Model file for the job. Use its own axes, mm. Give positions to 0.01 mm unless a question says otherwise; leave off trailing zeros. Order: outer loops, then holes, each group sorted by start corner. A loop starts at its lowest first (then second) coordinate and runs counter-clockwise, first axis right, second up. Notation, with made-up numbers: (24, 83) - (66, 83) arc R32 cw to (66, 118) - close; hole circle Ø8 at (79, -9). An arc over 180 degrees is marked (long way). Return JSON: item names as keys, results as strings. Group by question number.
from build123d import *

# Parameters (mm, degrees)
EXTRUDE_THIN2_DEPTH      = 2.25
EXTRUDE_THIN2_DEPTH_BACK = 2.25
SKETCH2_W                = 2.5
SKETCH2_H                = 0.8
EXTRUDE1_DEPTH           = 4
EXTRUDE1_DEPTH_BACK      = 4
S2D0010_W                = 0.5
S2D0010_H                = 2.5
EXTRUDE2_DEPTH           = 0.17
EXTRUDE_THIN3_DEPTH      = 0.5
EXTRUDE_THIN3_DEPTH_BACK = 0.5
FILLET1_R                = 0.15
FILLET2_R                = 0.49


with BuildPart() as part:
    # Sketch1 → Extrude-Thin2 (new body, two sides)
    with BuildSketch(Plane(origin=(0, 0, 0), x_dir=(0, -1, 0), z_dir=(1, 0, 0))) as extrude_thin2_sk:
        with BuildLine():
            Line((-3.4, -0.6), (-2.8, -0.6))
            ThreePointArc((-2.8, -0.6), (-2.693933983, -0.556066017), (-2.65, -0.45))
            Line((-2.65, -0.45), (-2.65, 0))
            Line((-2.65, 0), (2.65, 0))
            Line((2.65, 0), (2.65, -0.45))
            ThreePointArc((2.65, -0.45), (2.693933983, -0.556066017), (2.8, -0.6))
            Line((2.8, -0.6), (3.4, -0.6))
            Line((3.4, -0.6), (3.4, -0.5))
            Line((3.4, -0.5), (2.8, -0.5))
            ThreePointArc((2.8, -0.5), (2.764644661, -0.485355339), (2.75, -0.45))
            Line((2.75, -0.45), (2.75, 0.1))
            Line((2.75, 0.1), (-2.75, 0.1))
            Line((-2.75, 0.1), (-2.75, -0.45))
            ThreePointArc((-2.75, -0.45), (-2.764644661, -0.485355339), (-2.8, -0.5))
            Line((-2.8, -0.5), (-3.4, -0.5))
            Line((-3.4, -0.5), (-3.4, -0.6))
        make_face()
    extrude(amount=EXTRUDE_THIN2_DEPTH)
    extrude(extrude_thin2_sk.sketch, amount=-EXTRUDE_THIN2_DEPTH_BACK)

    # Sketch2 → Extrude1 (cut, two sides)
    with BuildSketch(Plane(origin=(0, 0, 0), x_dir=(-1, 0, 0), z_dir=(0, 1, 0))) as extrude1_sk:
        with Locations((0, 0.4)):
            Rectangle(SKETCH2_W, SKETCH2_H)
    extrude(amount=EXTRUDE1_DEPTH, mode=Mode.SUBTRACT)
    extrude(extrude1_sk.sketch, amount=-EXTRUDE1_DEPTH_BACK, mode=Mode.SUBTRACT)

    # S2D0010 → Extrude2 (cut)
    with BuildSketch(Plane(origin=(0, 0, 0), x_dir=(0, -1, 0), z_dir=(0, 0, 1))):
        with BuildLine():
            Line((1.25, 1), (-1.25, 1))
            ThreePointArc((-1.25, 1), (-2.25, 0), (-1.25, -1))
            Line((-1.25, -1), (1.25, -1))
            ThreePointArc((1.25, -1), (2.25, 0), (1.25, 1))
        make_face()
        with Locations((2.75, 0)):
            Rectangle(S2D0010_W, S2D0010_H)
        with Locations((-2.75, 0)):
            Rectangle(S2D0010_W, S2D0010_H)
    extrude(amount=-EXTRUDE2_DEPTH, mode=Mode.SUBTRACT)

    # S2D0012 → Extrude-Thin3 (add, two sides)
    with BuildSketch(Plane(origin=(0, 0, 0), x_dir=(1, 0, 0), z_dir=(0, 1, 0))) as extrude_thin3_sk:
        with BuildLine():
            Line((2.25, 0), (2.45, 0))
            ThreePointArc((2.45, 0), (2.485355339, -0.014644661), (2.5, -0.05))
            Line((2.5, -0.05), (2.5, -1.4))
            Line((2.5, -1.4), (2.6, -1.4))
            Line((2.6, -1.4), (2.6, -0.05))
            ThreePointArc((2.6, -0.05), (2.556066017, 0.056066017), (2.45, 0.1))
            Line((2.45, 0.1), (2.25, 0.1))
            Line((2.25, 0.1), (2.25, 0))
        make_face()
    extrude(amount=EXTRUDE_THIN3_DEPTH)
    extrude(extrude_thin3_sk.sketch, amount=-EXTRUDE_THIN3_DEPTH_BACK)

    # Fillet1
    fillet1_edges = [part.edges().sort_by_distance(p)[0] for p in [
        (-1.75, -2.75, -0.1),
    ]]
    fillet(fillet1_edges, radius=FILLET1_R)

    # Fillet2
    fillet2_edges = [part.edges().sort_by_distance(p)[0] for p in [
        (2.25, -3.4, 0.55),
    ]]
    fillet(fillet2_edges, radius=FILLET2_R)


solid = part.part
(1) Slice it at B-B (z = 0.3). Give the cut face in (x, y), and give its area (3 significant figures).
(2) Drop flat-ended pins along their axis: pin 1 Ø1 at (x, y) = (1, 0) entering from +Z; pin 2 Ø0.7 at (x, y) = (2, 3) entering from +Z; pin 3 Ø0.8 at (y, z) = (3, 0.5) entering from +X. Give the stop position or say it passes through.
(3) Slice it at A-A (y = -0.75). Give the cut face in (x, z), and give its area (3 significant figures).
(4) Slice it at C-C (x = 0). Give the cut face in (y, z).
(5) Slice it at D-D (x = -1.5). Give the cut face in (y, z).
Result set:
{
 "1": {"outline": "(-2.25, -2.75) - (-1.25, -2.75) - (-1.25, -2.65) - (-2.25, -2.65) - close; (-2.25, 2.65) - (-1.25, 2.65) - (-1.25, 2.75) - (-2.25, 2.75) - close; (1.25, -2.75) - (2.25, -2.75) - (2.25, -2.65) - (1.25, -2.65) - close; (1.25, 2.65) - (2.25, 2.65) - (2.25, 2.75) - (1.25, 2.75) - close; (2.5, -0.5) - (2.6, -0.5) - (2.6, 0.5) - (2.5, 0.5) - close", "area": "0.500 mm²"},
 "2": {"pin 1": "stops at z = 0", "pin 2": "stops at z = 0.6", "pin 3": "stops at x = 2.25"},
 "3": {"outline": "(-2.25, -0.1) - (-1, -0.1) - (-1, 0) - (-2.25, 0) - close; (1, -0.1) - (2.25, -0.1) - (2.25, 0) - (1, 0) - close", "area": "0.250 mm²"},
 "4": {"outline": "(-2.5, -0.1) - (-2.25, -0.1) - (-2.25, 0) - (-2.5, 0) - close; (2.25, -0.1) - (2.5, -0.1) - (2.5, 0) - (2.25, 0) - close"},
 "5": {"outline": "(-3.4, 0.5) - (-2.8, 0.5) arc R0.05 cw to (-2.75, 0.45) - (-2.75, 0.05) arc R0.15 ccw to (-2.6, -0.1) - (2.75, -0.1) - (2.75, 0.45) arc R0.05 cw to (2.8, 0.5) - (3.4, 0.5) - (3.4, 0.6) - (2.8, 0.6) arc R0.15 ccw to (2.65, 0.45) - (2.65, 0) - (-2.65, 0) - (-2.65, 0.45) arc R0.15 ccw to (-2.8, 0.6) - (-3.4, 0.6) - close"}
}
